Read the model definition and answer for the solid it produces. Units are mm, in the model's axes. A direction names the side the tool comes from. Coordinates: 2 decimals unless noted, no trailing zeros. Order: outer loops, then holes, each group sorted by start corner. A loop starts at its lowest first (then second) coordinate and runs counter-clockwise, first axis right, second up. Notation, with made-up numbers: M 39,-33.5 L 63,-33.5 A14 ccw 63,-21.5 Z; hole C 55,56 d5. An arc over 180 degrees is marked long. One line per question, with ' | ' between items. Start each with the question number.
1) Consider probe 1 along Z at (x, y) = (26, 0); probe 2 along Z at (x, y) = (-1.5, 1.5). Determine where each line is inside the solid, lowest interval first.
2) Given P1, Ø1.5, axis at x = 15, y = 1, coming from the -Z side; P2, Ø4, axis at x = 8.5, z = 0.5, coming from the +Y side, each flat-ended and moving along its own axis, determine where each tip first touches the part or whether it passes through.
3) Find section A-A, the plane x = 27. Write down the section's boundary in (y, z).
4) A tool of negligible diameter and unlimited length cuts with its end or side. For faces 1 (the face through (-0.646, -1.702, -1.561)), 2 (the face through (17.255, 1.797, -0.757)), 3 (the face through (17.255, -0.757, -1.797)), 4 (the face through (17.255, 0.757, 1.797)), from which of +Z, -Z, +X, -X, +Y, -Y can it reach the whole face along a straight path? Write none if from no direction.
from build123d import *

# Parameters (mm, degrees)
BOSS_EXTRUDE1_DEPTH = 35


with BuildPart() as part:
    # Sketch1 → Boss-Extrude1 (new body)
    with BuildSketch(Plane(origin=(0, 0, 0), x_dir=(0, 0, -1), z_dir=(1, 0, 0))):
        Polygon((-2.110664791, 0), (-1.492465386, -1.492465386), (0, -2.110664791), (1.492465386, -1.492465386), (2.110664791, 0), (1.492465386, 1.492465386), (0, 2.110664791), (-1.492465386, 1.492465386), align=None)
    extrude(amount=BOSS_EXTRUDE1_DEPTH)

    # Sketch4 → Revolve1 (revolve)
    with BuildSketch(Plane.XY):
        Polygon((0, 0), (-5, 0), (-5, 3.5), (-2.5, 3.5), (-1.309401077, 2.309401077), (0, 2.309401077), align=None)
    revolve(axis=Axis((0, 0, 0), (-1, 0, 0)))


solid = part.part
Report:
1) probe 1: z = -2.11 to 2.11 | probe 2: z = -2 to 2
2) P1: stops at z = -2.01 | P2: stops at y = 2.11
3) outline: M -2.11,0 L -1.49,-1.49 L 0,-2.11 L 1.49,-1.49 L 2.11,0 L 1.49,1.49 L 0,2.11 L -1.49,1.49 Z
4) face 1: +X | face 2: -Z, +X, +Y | face 3: -Z, +X, -Y | face 4: +Z, +X, +Y
